Read the model definition and answer for the solid it produces. Units are mm, in the model's axes. A direction names the side the tool comes from. Give positions to 0.01 mm unless a question says otherwise; leave off trailing zeros. Loops run counter-clockwise (first coordinate to the right, second up) from the corner with the lowest first, then second, coordinate; pieces in that order, holes last.
(1) Find section D-D, the plane z = 14.5. Write down the section's boundary in (x, y).
(2) Determine the mould class of faces 1 (the face through (25.02, 15.57, 16)), 2 (the face through (25.93, 0.35, 0.6)), 3 (the face through (2, 12.094, 2)) for opening direction X: pulls with the +X half, pulls with the -X half, needs draft (parallel to the pull), parting line crosses it, or undercut.
(3) Straight lines are drawn through the part: probe 1 along Y at (x, z) = (25.3, 14.5); probe 2 along Y at (x, z) = (25.6, 30); probe 3 along X at (y, z) = (-22, 38). For each, find the intervals that lie inside material, in ascending order.
(4) Find section A-A, the plane x = -10. Write down the section's boundary in (y, z), then the cut area to 3 significant figures.
(5) Each of these flat-tipped pins is pushed along its axis until it touches: P1, Ø6, axis at y = 2.5, z = 19.5, coming from the -X side; P2, Ø2, axis at x = -21, y = -4, coming from the +Z side. Where does it stop, or does it pass through?
(6) Find section C-C, the plane z = 30. Write down the section's boundary in (x, y), then the cut area to 3 significant figures.
(7) Which of the six approach directions +Z, -Z, +X, -X, +Y, -Y give full straight-line access (tool end or side, diameter ignored) to faces 4 (the face through (26.5, 0, 15)), 5 (the face through (-16.27, -15.52, 1.52)), 6 (the face through (19, 22, 8))?
(8) Find section B-B, the plane y = 0. Write down the section's boundary in (x, z), then the cut area to 3 significant figures.
```python
from build123d import *

# Parameters (mm, degrees)
SZKIC5_W                    = 53
SZKIC5_H                    = 50
DODANIE_WYCI_GNI_CIE2_DEPTH = 3
SZKIC6_W                    = 3
SZKIC6_H                    = 50
DODANIE_WYCI_GNI_CIE3_DEPTH = 48
ZAOKR_GLENIE1_R             = 2
SFAZOWANIE2_SIZE            = 3
SFAZOWANIE4_SIZE            = 3
WYTNIJ_WYCI_GNI_CIE2_REACH  = 79.685
SZKIC7_R                    = 11.05
WYTNIJ_WYCI_GNI_CIE3_REACH  = 79.685
SZKIC9_R                    = 1.5
WYTNIJ_WYCI_GNI_CIE4_REACH  = 79.685
SZKIC10_R                   = 1.5
WYTNIJ_WYCI_GNI_CIE5_REACH  = 79.685
SZKIC11_R                   = 1.5
WYTNIJ_WYCI_GNI_CIE6_REACH  = 79.685
SZKIC12_R                   = 1.5
DODANIE_WYCI_GNI_CIE4_DEPTH = 3
DODANIE_WYCI_GNI_CIE5_DEPTH = 3
WYTNIJ_WYCI_GNI_CIE7_DEPTH  = 3


with BuildPart() as part:
    # Szkic5 → Dodanie-wyciągnięcie2 (new body)
    with BuildSketch(Plane.XY):
        Rectangle(SZKIC5_W, SZKIC5_H)
    extrude(amount=DODANIE_WYCI_GNI_CIE2_DEPTH)

    # Szkic6 → Dodanie-wyciągnięcie3 (add)
    with BuildSketch(Plane.XY.offset(3)):
        with Locations((25, 0)):
            Rectangle(SZKIC6_W, SZKIC6_H)
    extrude(amount=DODANIE_WYCI_GNI_CIE3_DEPTH)

    # Zaokrąglenie1
    zaokr_glenie1_edges = [part.edges().sort_by_distance(p)[0] for p in [
        (26.5, 0, 0),
    ]]
    fillet(zaokr_glenie1_edges, radius=ZAOKR_GLENIE1_R)

    # Sfazowanie2
    sfazowanie2_edges = [part.edges().sort_by_distance(p)[0] for p in [
        (25, -25, 51),
        (-26.5, -25, 1.5),
        (-26.5, 25, 1.5),
    ]]
    chamfer(sfazowanie2_edges, length=SFAZOWANIE2_SIZE)

    # Sfazowanie4
    sfazowanie4_edges = [part.edges().sort_by_distance(p)[0] for p in [
        (25, 25, 51),
    ]]
    chamfer(sfazowanie4_edges, length=SFAZOWANIE4_SIZE)

    # Szkic7 → Wytnij-wyciągnięcie2 (cut, up to next)
    with BuildSketch(Plane(origin=(26.5, 0, 0), x_dir=(0, 0, -1), z_dir=(1, 0, 0)), mode=Mode.PRIVATE) as wytnij_wyci_gni_cie2_sk1:
        with Locations((-30, 0)):
            Circle(SZKIC7_R)
    wytnij_wyci_gni_cie2_tool1 = extrude(wytnij_wyci_gni_cie2_sk1.sketch, amount=-WYTNIJ_WYCI_GNI_CIE2_REACH, mode=Mode.PRIVATE) & part.part
    add(wytnij_wyci_gni_cie2_tool1.solids().sort_by_distance((26.5, 0, 30))[0], mode=Mode.SUBTRACT)

    # Szkic9 → Wytnij-wyciągnięcie3 (cut, up to next)
    with BuildSketch(Plane(origin=(26.5, 0, 0), x_dir=(0, 0, -1), z_dir=(1, 0, 0)), mode=Mode.PRIVATE) as wytnij_wyci_gni_cie3_sk1:
        with Locations((-45.5, 15.5)):
            Circle(SZKIC9_R)
    wytnij_wyci_gni_cie3_tool1 = extrude(wytnij_wyci_gni_cie3_sk1.sketch, amount=-WYTNIJ_WYCI_GNI_CIE3_REACH, mode=Mode.PRIVATE) & part.part
    add(wytnij_wyci_gni_cie3_tool1.solids().sort_by_distance((26.5, 15.5, 45.5))[0], mode=Mode.SUBTRACT)

    # Szkic10 → Wytnij-wyciągnięcie4 (cut, up to next)
    with BuildSketch(Plane(origin=(26.5, 0, 0), x_dir=(0, 0, -1), z_dir=(1, 0, 0)), mode=Mode.PRIVATE) as wytnij_wyci_gni_cie4_sk1:
        with Locations((-45.5, -15.5)):
            Circle(SZKIC10_R)
    wytnij_wyci_gni_cie4_tool1 = extrude(wytnij_wyci_gni_cie4_sk1.sketch, amount=-WYTNIJ_WYCI_GNI_CIE4_REACH, mode=Mode.PRIVATE) & part.part
    add(wytnij_wyci_gni_cie4_tool1.solids().sort_by_distance((26.5, -15.5, 45.5))[0], mode=Mode.SUBTRACT)

    # Szkic11 → Wytnij-wyciągnięcie5 (cut, up to next)
    with BuildSketch(Plane(origin=(26.5, 0, 0), x_dir=(0, 0, -1), z_dir=(1, 0, 0)), mode=Mode.PRIVATE) as wytnij_wyci_gni_cie5_sk1:
        with Locations((-14.5, -15.5)):
            Circle(SZKIC11_R)
    wytnij_wyci_gni_cie5_tool1 = extrude(wytnij_wyci_gni_cie5_sk1.sketch, amount=-WYTNIJ_WYCI_GNI_CIE5_REACH, mode=Mode.PRIVATE) & part.part
    add(wytnij_wyci_gni_cie5_tool1.solids().sort_by_distance((26.5, -15.5, 14.5))[0], mode=Mode.SUBTRACT)

    # Szkic12 → Wytnij-wyciągnięcie6 (cut, up to next)
    with BuildSketch(Plane(origin=(26.5, 0, 0), x_dir=(0, 0, -1), z_dir=(1, 0, 0)), mode=Mode.PRIVATE) as wytnij_wyci_gni_cie6_sk1:
        with Locations((-14.5, 15.5)):
            Circle(SZKIC12_R)
    wytnij_wyci_gni_cie6_tool1 = extrude(wytnij_wyci_gni_cie6_sk1.sketch, amount=-WYTNIJ_WYCI_GNI_CIE6_REACH, mode=Mode.PRIVATE) & part.part
    add(wytnij_wyci_gni_cie6_tool1.solids().sort_by_distance((26.5, 15.5, 14.5))[0], mode=Mode.SUBTRACT)

    # Szkic15 → Dodanie-wyciągnięcie4 (add)
    with BuildSketch(Plane(origin=(0, 25, 0), x_dir=(1, 0, 0), z_dir=(0, 1, 0))):
        Polygon((23.5, -16), (10.5, -3), (23.5, -3), align=None)
    extrude(amount=-DODANIE_WYCI_GNI_CIE4_DEPTH)

    # Szkic16 → Dodanie-wyciągnięcie5 (add)
    with BuildSketch(Plane.XZ.offset(25)):
        Polygon((23.5, 3), (23.5, 16), (10.5, 3), align=None)
    extrude(amount=-DODANIE_WYCI_GNI_CIE5_DEPTH)

    # Szkic17 → Wytnij-wyciągnięcie7 (cut)
    with BuildSketch(Plane.XY.offset(3)):
        with BuildLine():
            Line((16.551792378, 12.093759381), (-13.448207622, 12.093759381))
            ThreePointArc((-13.448207622, 12.093759381), (-15.548207622, 14.193759381), (-13.448207622, 16.293759381))
            Line((-13.448207622, 16.293759381), (16.551792378, 16.293759381))
            ThreePointArc((16.551792378, 16.293759381), (18.651792378, 14.193759381), (16.551792378, 12.093759381))
        make_face()
        with BuildLine():
            Line((15.82894882, -17.577234295), (-14.17105118, -17.577234295))
            ThreePointArc((-14.17105118, -17.577234295), (-16.27105118, -15.477234295), (-14.17105118, -13.377234295))
            Line((-14.17105118, -13.377234295), (15.82894882, -13.377234295))
            ThreePointArc((15.82894882, -13.377234295), (17.92894882, -15.477234295), (15.82894882, -17.577234295))
        make_face()
    extrude(amount=-WYTNIJ_WYCI_GNI_CIE7_DEPTH, mode=Mode.SUBTRACT)


solid = part.part
```
Entries:
1. outline: (22, -25) - (26.5, -25) - (26.5, -17) - (23.5, -17) - (23.5, -22) - (22, -22) - close; (22, 22) - (23.5, 22) - (23.5, 17) - (26.5, 17) - (26.5, 25) - (22, 25) - close; (23.5, -14) - (26.5, -14) - (26.5, 14) - (23.5, 14) - close
2. face 1: needs draft
2. face 2: pulls with the +X half
2. face 3: undercut
3. probe 1: y = -25 to -17, -14 to 14, 17 to 25
3. probe 2: y = -25 to -11.05, 11.05 to 25
3. probe 3: x = 23.5 to 26.5
4. outline: (-25, 0) - (-17.58, 0) - (-17.58, 3) - (-25, 3) - close; (-13.38, 0) - (12.09, 0) - (12.09, 3) - (-13.38, 3) - close; (16.29, 0) - (25, 0) - (25, 3) - (16.29, 3) - close
4. area: 125 mm2
5. P1: stops at x = 23.5
5. P2: stops at z = 3
6. outline: (23.5, -25) - (26.5, -25) - (26.5, -11.05) - (23.5, -11.05) - close; (23.5, 11.05) - (26.5, 11.05) - (26.5, 25) - (23.5, 25) - close
6. area: 83.7 mm2
7. face 4: +Z, -Z, +X, +Y, -Y
7. face 5: +Z, -Z
7. face 6: +Z, -X
8. outline: (-26.5, 0) - (24.5, 0) arc R2 ccw to (26.5, 2) - (26.5, 18.95) - (23.5, 18.95) - (23.5, 3) - (-26.5, 3) - close; (23.5, 41.05) - (26.5, 41.05) - (26.5, 51) - (23.5, 51) - close
8. area: 236 mm2
